Design review of the part built by this model. Coordinates are the model's own, in mm. A direction names the side the tool comes from. Give positions to 0.01 mm unless a question says otherwise; leave off trailing zeros. Loops run counter-clockwise (first coordinate to the right, second up) from the corner with the lowest first, then second, coordinate; pieces in that order, holes last.
from build123d import *

# Parameters (mm, degrees)
SKETCH1_R           = 2.5
BOSS_EXTRUDE1_DEPTH = 5
BOSS_EXTRUDE2_START = 5
SKETCH1_3_R         = 4
BOSS_EXTRUDE2_DEPTH = 1
BOSS_EXTRUDE3_START = 6
SKETCH1_4_R         = 4
SKETCH1_4_R_2       = 3
BOSS_EXTRUDE3_DEPTH = 29


with BuildPart() as part:
    # Sketch1 → Boss-Extrude1 (new body)
    with BuildSketch(Plane(origin=(0, 0, 0), x_dir=(1, 0, 0), z_dir=(0, 1, 0))):
        Circle(SKETCH1_R)
    extrude(amount=BOSS_EXTRUDE1_DEPTH)

    # Sketch1<3> → Boss-Extrude2 (add)
    with BuildSketch(Plane(origin=(0, 0, 0), x_dir=(1, 0, 0), z_dir=(0, 1, 0)).offset(BOSS_EXTRUDE2_START)):
        Circle(SKETCH1_3_R)
    extrude(amount=BOSS_EXTRUDE2_DEPTH)

    # Sketch1<4> → Boss-Extrude3 (add)
    with BuildSketch(Plane(origin=(0, 0, 0), x_dir=(1, 0, 0), z_dir=(0, 1, 0)).offset(BOSS_EXTRUDE3_START)):
        Circle(SKETCH1_4_R)
        Circle(SKETCH1_4_R_2, mode=Mode.SUBTRACT)
    extrude(amount=BOSS_EXTRUDE3_DEPTH)


solid = part.part
Q1. Insertion check: pin 1 (2 mm diameter, centred on y = 17, z = -2.5, fed in from -X); pin 2 (2 mm diameter, centred on y = 16.5, z = -1.5, fed in from -X); pin 3 (2 mm diameter, centred on y = 15.5, z = -3, fed in from +X). Each pin has a flat end and moves straight along its axis. Give the tip position at first contact, or say it passes through.
Results:
pin 1: stops at x = -3.71
pin 2: stops at x = -3.97
pin 3: stops at x = 3.46
Q2. Take a section at D-D (y = 3). Give the boundary of the cut face in (x, z), plus the area to 3 significant figures.
Results:
outline: circle Ø5 at (0, 0)
area: 19.6 mm2
Q3. Take a section at B-B (y = 10). Give the boundary of the cut face in (x, z).
Results:
outline: circle Ø8 at (0, 0); hole circle Ø6 at (0, 0)
Q4. Wall thickness on line 1 (X direction, y = 25, z = 0); line 2 (Y direction, x = 2.25, z = 2.5): over which ranges is each line inside the solid? List them lowest first.
Results:
line 1: x = -4 to -3, 3 to 4
line 2: y = 5 to 35
Q5. Take a section at C-C (z = 1.75). Give the boundary of the cut face in (x, y).
Results:
outline: (-3.6, 5) - (-1.79, 5) - (-1.79, 0) - (1.79, 0) - (1.79, 5) - (3.6, 5) - (3.6, 35) - (2.44, 35) - (2.44, 6) - (-2.44, 6) - (-2.44, 35) - (-3.6, 35) - close
Q6. Take a section at A-A (x = 0). Give the boundary of the cut face in (y, z).
Results:
outline: (0, -2.5) - (5, -2.5) - (5, -4) - (35, -4) - (35, -3) - (6, -3) - (6, 3) - (35, 3) - (35, 4) - (5, 4) - (5, 2.5) - (0, 2.5) - close
Q7. Draft analysis for pull direction X (two halves, no side actions). For faces 4 (the face through (2, 5, -2)), 5 (the face through (-3, 20, 0)), 6 (the face through (-0.867, 19.79, 3.905)), state which applies: pulls with the +X half, pulls with the -X half, needs draft (parallel to the pull), parting line crosses it, or undercut.
Results:
face 4: needs draft
face 5: undercut
face 6: parting line crosses it
Q8. Tool access review of faces 1 (the face through (0, 0, 0)), 2 (the face through (-0.54, 2.46, 2.44)), 3 (the face through (0, 6, 0)): name each direction out of +Z, -Z, +X, -X, +Y, -Y from which nothing blocks a thin tool from reaching the whole face with its end or side.
Results:
face 1: +Z, -Z, +X, -X, -Y
face 2: -Y
face 3: +Y
